Can you work these out from the model? Positions are in its coordinate system, mm. Coordinates: 2 decimals unless noted, no trailing zeros. Order: outer loops, then holes, each group sorted by start corner. A loop starts at its lowest first (then second) coordinate and runs counter-clockwise, first axis right, second up. Notation, with made-up numbers: M -15.5,-7.5 L 12.5,-7.5 A14 cw 12.5,-1.5 Z; hole C 6,21.25 d11. An arc over 180 degrees is marked long. Answer as a JSON object with one key per item and string values.
from build123d import *

# Parameters (mm, degrees)
BOX003_W     = 115
BOX003_H     = 5
BOX003_DEPTH = 115
FILLET003_R  = 23
BOX002_W     = 127
BOX002_H     = 5
BOX002_DEPTH = 127
FILLET002_R  = 26


with BuildPart() as inside001:
    # Box003 → Box003 (new body)
    with BuildSketch(Plane(origin=(-57.5, 20, -57.5), x_dir=(1, 0, 0), z_dir=(0, 0, 1))):
        with Locations((57.5, 2.5)):
            Rectangle(BOX003_W, BOX003_H)
    extrude(amount=BOX003_DEPTH)

    # Fillet003
    fillet003_edges = [inside001.edges().sort_by_distance(p)[0] for p in [
        (-57.5, 22.5, 57.5),
        (-57.5, 22.5, -57.5),
        (57.5, 22.5, 57.5),
        (57.5, 22.5, -57.5),
    ]]
    fillet(fillet003_edges, radius=FILLET003_R)


with BuildPart() as cover:
    # Box002 → Box002 (new body)
    with BuildSketch(Plane(origin=(-63.5, 25, -63.5), x_dir=(1, 0, 0), z_dir=(0, 0, 1))):
        with Locations((63.5, 2.5)):
            Rectangle(BOX002_W, BOX002_H)
    extrude(amount=BOX002_DEPTH)

    # Fillet002
    fillet002_edges = [cover.edges().sort_by_distance(p)[0] for p in [
        (-63.5, 27.5, 63.5),
        (-63.5, 27.5, -63.5),
        (63.5, 27.5, 63.5),
        (63.5, 27.5, -63.5),
    ]]
    fillet(fillet002_edges, radius=FILLET002_R)

    # Fusion: union Inside001
    add(inside001.part)


with BuildPart() as cover_1:
    # Fusion placement: moved
    add(cover.part.moved(Location((0, 18, 0))))


solid = cover_1.part
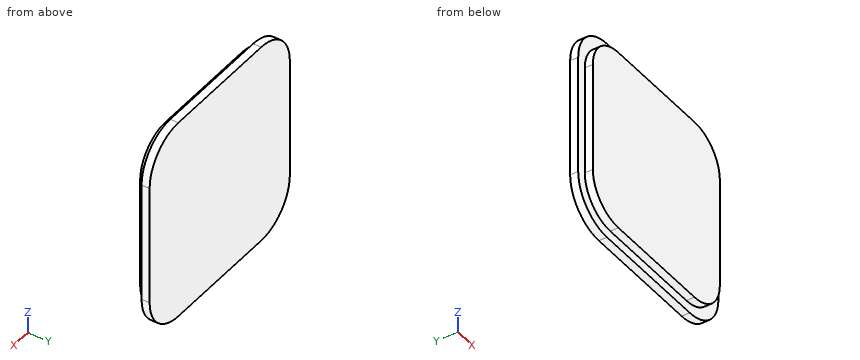
Item 1: I want a section at B-B, the plane z = -31.5. Write out the boundary of the cut face in (x, y), plus the area to 3 significant figures.
Answers follow:
{"outline": "M -63.5,43 L -57.5,43 L -57.5,38 L 57.5,38 L 57.5,43 L 63.5,43 L 63.5,48 L -63.5,48 Z", "area": "1,210 mm^2"}
Item 2: Please list where these lines run through material, in increasing order: line 1 (Z direction, x = -6, y = 39.25); line 2 (X direction, y = 45.25, z = 40).
Answers follow:
{"line 1": "z = -57.5 to 57.5", "line 2": "x = -63.38 to 63.38"}
Item 3: I want a section at A-A, the plane y = 46. Write out the boundary of the cut face in (x, z).
Answers follow:
{"outline": "M -63.5,-37.5 A26 ccw -37.5,-63.5 L 37.5,-63.5 A26 ccw 63.5,-37.5 L 63.5,37.5 A26 ccw 37.5,63.5 L -37.5,63.5 A26 ccw -63.5,37.5 Z"}
Item 4: I'm going to push flat-ended pins straight in: pin 1 (2.5 mm diameter, centred on y = 40, z = 6, fed in from +X); pin 2 (5.5 mm diameter, centred on y = 40, z = -7, fed in from -X); pin 3 (1.5 mm diameter, centred on x = 7.5, y = 41, fed in from -Z). Where does each tip first touch, or does it pass through?
Answers follow:
{"pin 1": "stops at x = 57.5", "pin 2": "stops at x = -57.5", "pin 3": "stops at z = -57.5"}
